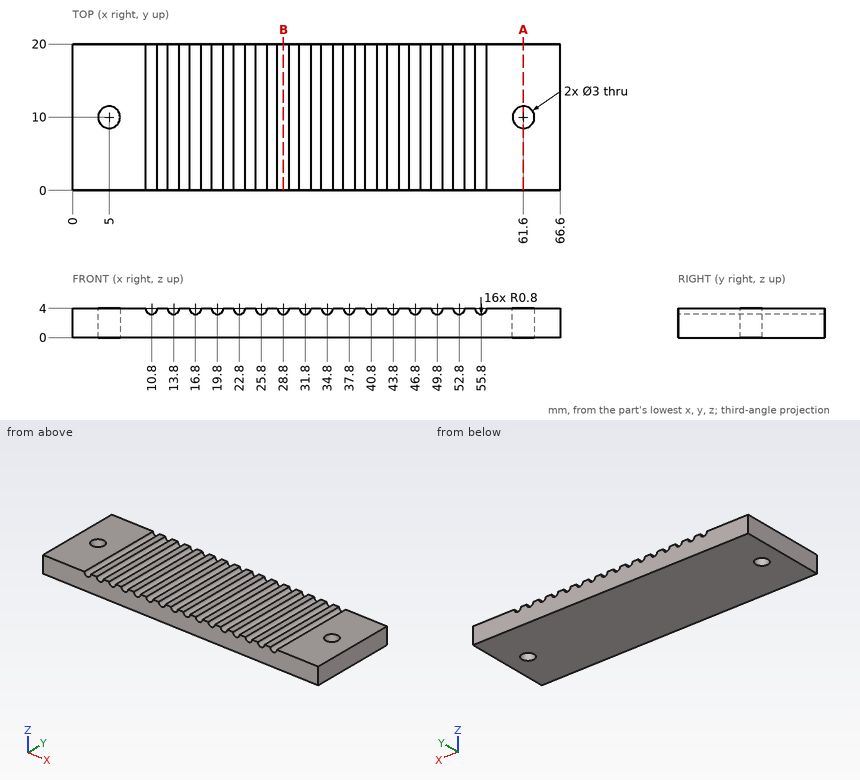
Design review of the part shown in the three views and the two pictorial views. Dimensions are in mm from the part's minimum x, y and z. Round coordinates to 2 decimals unless told otherwise and drop trailing zeros. Order: outer loops, then holes, each group sorted by start corner. A loop starts at its lowest first (then second) coordinate and runs counter-clockwise, first axis right, second up. Notation, with made-up numbers: M 41,31 L 91,31 A14 cw 91,39 Z; hole C 73.25,70.25 d1. An arc over 180 degrees is marked long. Put each result on its own line as item: value.
Q1. Consider section A-A (x = 61.6). State the section outline as (y, z) points.
Reported:
outline: M 0,0 L 8.5,0 L 8.5,4 L 0,4 Z; M 11.5,0 L 20,0 L 20,4 L 11.5,4 Z
Q2. To check wall thickness, follow line 1 (Y direction, x = 61.6, z = 2.5); line 2 (Z direction, x = 53, y = 2.75); line 3 (Z direction, x = 47.5, y = 9). State the ranges of each line that lie inside material, in increasing order.
Reported:
line 1: 0 to 8.5, 11.5 to 20
line 2: 0 to 3.23
line 3: 0 to 3.61
Q3. Consider section B-B (x = 28.8). State the section outline as (y, z) points, and give its area (3 significant figures).
Reported:
outline: M 0,0 L 20,0 L 20,3.2 L 0,3.2 Z
area: 64.0 mm²
Q4. Insertion check: pin 1 Ø2.5 at (x, y) = (5, 10) entering from -Z; pin 2 Ø6 at (x, y) = (39, 13) entering from -Z. Each pin has a flat end and moves straight along its axis. Give the tip position at first contact, or say it passes through.
Reported:
pin 1: through
pin 2: z = 0
